Can you work these out from the drawing? Everything is in mm from the part's minimum corner. Give positions to 0.01 mm unless a question says otherwise; leave off trailing zeros. Loops run counter-clockwise (first coordinate to the right, second up) from the corner with the lowest first, then second, coordinate; pieces in that order, holes last. Notation, with made-up numbers: (73.25, 44.25) -> (84.25, 44.25) arc R18 ccw to (84.25, 64.25) -> close; hole circle Ø2 at (19.5, -39). An arc over 180 degrees is marked (long way). Write item = value, one per line. Start each with the question number.
1) I want a section at A-A (z = 2.5). List the corners of the cut face in (x, y) for me (1 decimal).
2) I need wall thicknesses on probe 1 along X at (y, z) = (90, 2); probe 2 along Y at (x, z) = (91, 0.5). Which ranges of each line are inside material? Lowest first, please. Write a range as from..to.
3) I want a section at B-B (x = 90). List the corners of the cut face in (y, z) for me.
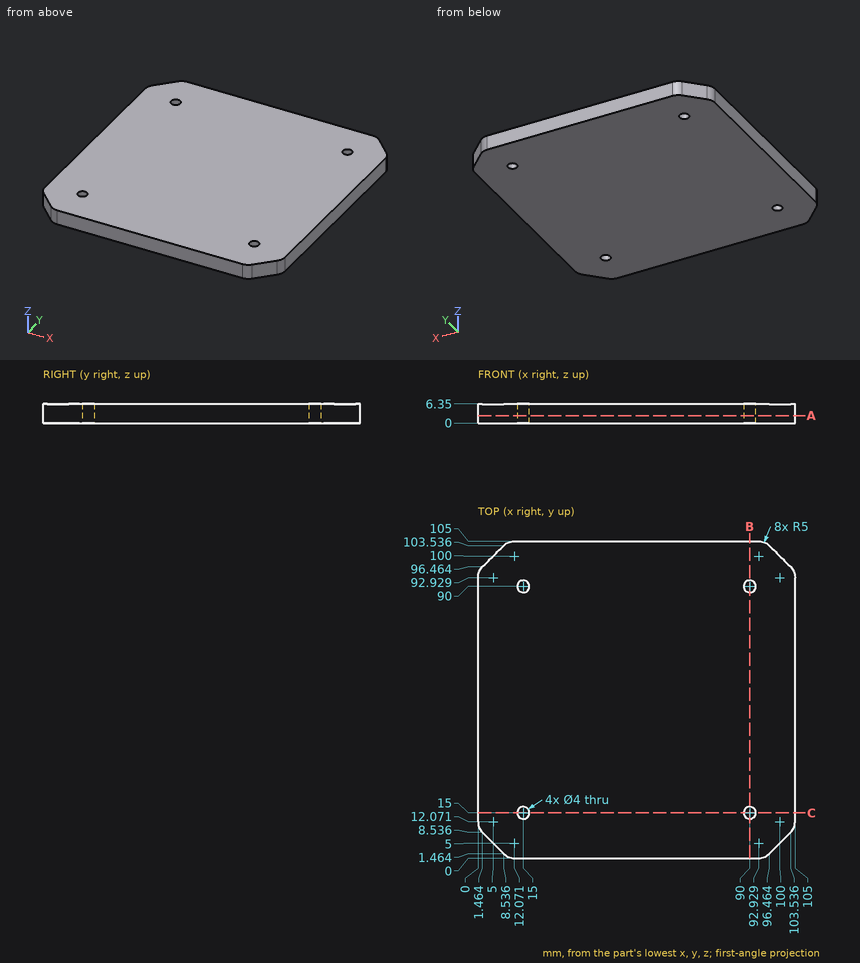
Answer list:
q1.outline = (0, 12.1) arc R5 ccw to (1.5, 8.5) -> (8.5, 1.5) arc R5 ccw to (12.1, 0) -> (92.9, 0) arc R5 ccw to (96.5, 1.5) -> (103.5, 8.5) arc R5 ccw to (105, 12.1) -> (105, 92.9) arc R5 ccw to (103.5, 96.5) -> (96.5, 103.5) arc R5 ccw to (92.9, 105) -> (12.1, 105) arc R5 ccw to (8.5, 103.5) -> (1.5, 96.5) arc R5 ccw to (0, 92.9) -> close; hole circle Ø4 at (15, 15); hole circle Ø4 at (15, 90); hole circle Ø4 at (90, 15); hole circle Ø4 at (90, 90)
q2.probe_1 = 0..13, 17..88, 92..105
q2.probe_2 = 0..13.27, 16.73..88.27, 91.73..105
q3.outline = (0, 0) -> (13, 0) -> (13, 6.35) -> (0, 6.35) -> close; (17, 0) -> (88, 0) -> (88, 6.35) -> (17, 6.35) -> close; (92, 0) -> (105, 0) -> (105, 6.35) -> (92, 6.35) -> close
